For this review, use the dimensioned drawing (mm, ordinates from the lowest corner) and the shaded views. A direction names the side the tool comes from. Coordinates: 2 decimals unless noted, no trailing zeros. Order: outer loops, then holes, each group sorted by start corner. A loop starts at its lowest first (then second) coordinate and runs counter-clockwise, first axis right, second up. Notation, with made-up numbers: M 66.25,74.5 L 97.25,74.5 A30 ccw 97.25,110.5 Z; hole C 50.25,28 d2. An arc over 180 degrees is marked long. Answer in a Markdown table with one row per item.
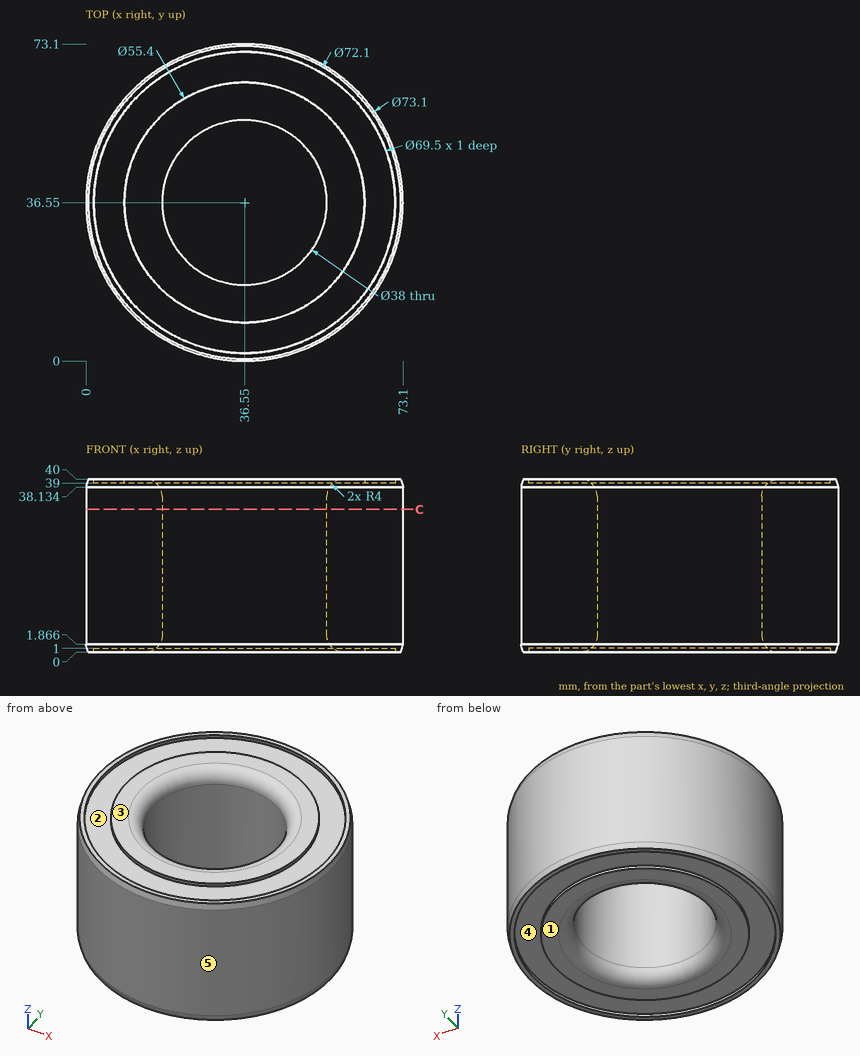
(1) For line 1 along Y through (x, z) = (36.55, 0.7); line 2 along Z through (x, y) = (68.5, 43.5); line 3 along Y through (x, z) = (33, 8), list the stretches that pass through material, from the lowest coordinate up. Write a range as from..to.
Return value:
| item | result |
|---|---|
| line 1 | y = 0.31..1.8, 8.85..15.81, 57.29..64.25, 71.3..72.79 |
| line 2 | z = 1..39 |
| line 3 | y = 0.17..17.88, 55.22..72.93 |
(2) Insertion check: pin 1 Ø8 at (x, z) = (10.5, 29.5) entering from +Y; pin 2 Ø1 at (x, z) = (29, 20) entering from +Y; pin 3 Ø3 at (y, z) = (62, 5) entering from +X; pin 4 Ø6 at (x, y) = (31, 16.5) entering from -Z. Each pin has a flat end and moves straight along its axis. Give the tip position at first contact, or say it passes through.
Return value:
| item | result |
|---|---|
| pin 1 | stops at y = 65.7 |
| pin 2 | stops at y = 72.41 |
| pin 3 | stops at x = 64.16 |
| pin 4 | stops at z = 0 |
(3) For the marked faces 1 and 2, list the 3-axis set-ups (+Z, -Z, +X, -X, +Y, -Y) from which the entire face can be reached by the end or side of a thin tool; tool diameter is ignored.
Return value:
| item | result |
|---|---|
| face 1 | -Z, +X, -X, +Y, -Y |
| face 2 | +Z |
(4) Draft analysis for pull direction Y (two halves, no side actions). For the marked faces 3, 4 and 5, state which applies: pulls with the +Y half, pulls with the -Y half, needs draft (parallel to the pull), parting line crosses it, or undercut.
Return value:
| item | result |
|---|---|
| face 3 | needs draft |
| face 4 | undercut |
| face 5 | parting line crosses it |
(5) Add section C-C, the plane z = 33. Give the boundary of the cut face in (x, y), and give its area (3 significant figures).
Return value:
| item | result |
|---|---|
| outline | C 36.55,36.55 d73.1; hole C 36.55,36.55 d38 |
| area | 3,060 mm2 |
